Could you check a few things on this model? Use its own coordinates, in mm. Give positions to 0.01 mm unless a question says otherwise; leave off trailing zeros. Write each loop counter-clockwise with the first axis right and the second up, starting at its lowest first coordinate (ties: lowest second). Pieces come first, ordered by that corner, then holes. Notation, with made-up numbers: (-13.5, 8.5) -> (35.5, 8.5) arc R7 ccw to (35.5, 13.5) -> close; hole circle Ø1 at (24.25, -24). An arc over 180 degrees is marked (long way). Write item = value, one per line. Start each with the question number.
```python
from build123d import *

# Parameters (mm, degrees)
SKETCH_1_W      = 26.5
SKETCH_1_H      = 21
SKETCH_1_R      = 0.4
EXTRUDE_1_DEPTH = 1.6
SKETCH_2_W      = 5.5
SKETCH_2_H      = 10
EXTRUDE_2_DEPTH = 1.6


with BuildPart() as part:
    # Эскиз1 → Бобышка-Вытянуть1 (new body)
    with BuildSketch(Plane.XY):
        Rectangle(SKETCH_1_W, SKETCH_1_H)
        with Locations((-11.43, -9)):
            Circle(SKETCH_1_R, mode=Mode.SUBTRACT)
        with Locations((-8.89, -9)):
            Circle(SKETCH_1_R, mode=Mode.SUBTRACT)
        with Locations((-6.35, -9)):
            Circle(SKETCH_1_R, mode=Mode.SUBTRACT)
        with Locations((-3.81, -9)):
            Circle(SKETCH_1_R, mode=Mode.SUBTRACT)
        with Locations((-1.27, -9)):
            Circle(SKETCH_1_R, mode=Mode.SUBTRACT)
        with Locations((1.27, -9)):
            Circle(SKETCH_1_R, mode=Mode.SUBTRACT)
        with Locations((3.81, -9)):
            Circle(SKETCH_1_R, mode=Mode.SUBTRACT)
        with Locations((6.35, -9)):
            Circle(SKETCH_1_R, mode=Mode.SUBTRACT)
        with Locations((8.89, -9)):
            Circle(SKETCH_1_R, mode=Mode.SUBTRACT)
        with Locations((11.43, -9)):
            Circle(SKETCH_1_R, mode=Mode.SUBTRACT)
        with Locations((-11.43, 9)):
            Circle(SKETCH_1_R, mode=Mode.SUBTRACT)
        with Locations((-8.89, 9)):
            Circle(SKETCH_1_R, mode=Mode.SUBTRACT)
        with Locations((-6.35, 9)):
            Circle(SKETCH_1_R, mode=Mode.SUBTRACT)
        with Locations((-3.81, 9)):
            Circle(SKETCH_1_R, mode=Mode.SUBTRACT)
        with Locations((-1.27, 9)):
            Circle(SKETCH_1_R, mode=Mode.SUBTRACT)
        with Locations((1.27, 9)):
            Circle(SKETCH_1_R, mode=Mode.SUBTRACT)
        with Locations((3.81, 9)):
            Circle(SKETCH_1_R, mode=Mode.SUBTRACT)
        with Locations((6.35, 9)):
            Circle(SKETCH_1_R, mode=Mode.SUBTRACT)
        with Locations((8.89, 9)):
            Circle(SKETCH_1_R, mode=Mode.SUBTRACT)
        with Locations((11.43, 9)):
            Circle(SKETCH_1_R, mode=Mode.SUBTRACT)
        with Locations((-8.89, 6.46)):
            Circle(SKETCH_1_R, mode=Mode.SUBTRACT)
        with Locations((-6.35, 6.46)):
            Circle(SKETCH_1_R, mode=Mode.SUBTRACT)
        with Locations((-3.81, 6.46)):
            Circle(SKETCH_1_R, mode=Mode.SUBTRACT)
        with Locations((-1.27, 6.46)):
            Circle(SKETCH_1_R, mode=Mode.SUBTRACT)
        with Locations((1.27, 6.46)):
            Circle(SKETCH_1_R, mode=Mode.SUBTRACT)
        with Locations((3.81, 6.46)):
            Circle(SKETCH_1_R, mode=Mode.SUBTRACT)
        with Locations((6.35, 6.46)):
            Circle(SKETCH_1_R, mode=Mode.SUBTRACT)
        with Locations((8.89, 6.46)):
            Circle(SKETCH_1_R, mode=Mode.SUBTRACT)
        with Locations((11.43, 6.46)):
            Circle(SKETCH_1_R, mode=Mode.SUBTRACT)
        with Locations((-11.43, 6.46)):
            Circle(SKETCH_1_R, mode=Mode.SUBTRACT)
    extrude(amount=EXTRUDE_1_DEPTH)

    # Эскиз2 → Бобышка-Вытянуть2 (add)
    with BuildSketch(Plane.XY.offset(1.6)):
        Rectangle(SKETCH_2_W, SKETCH_2_H)
    extrude(amount=EXTRUDE_2_DEPTH)


solid = part.part
```
(1) We'd pull the mould along Y, two halves only. Please class faces 1 (the flat face through (0, -10.5, 1)), 2 (the flat face through (2.75, 0, 2)), 3 (the cylindrical face through (11.11, -9.24, 0.79)): released by +Y, released by -Y, zero draft, split by the parting line, or undercut.
(2) Imagine slicing it at C-C (y = 6.46). State how many separate pieces and enclosed holes the cut face has, then the cut area to 3 significant figures.
(3) Imagine slicing it at A-A (x = -8.89). Please give me the cut outline in (y, z).
(4) I'm going to push flat-ended pins straight in: pin 1 (0.8 mm diameter, centred on y = 1.5, z = 2.5, fed in from -X); pin 2 (1.3 mm diameter, centred on x = 1, z = 2, fed in from -Y); pin 3 (12 mm diameter, centred on x = 10, y = -4, fed in from +Z); pin 4 (1.5 mm diameter, centred on y = -3.5, z = 2.5, fed in from +X). Where does each tip first touch, or does it pass through?
(5) Imagine slicing it at B-B (x = 2.25). Please give me the cut outline in (y, z).
(6) If I drill on line 1 along Y through (x, z) = (-6.35, 0.55); line 2 along Y through (x, z) = (1, 1.1); line 3 along Z through (x, y) = (-7, -7.5), over which ranges is the centre line in solid material (lowest first)? Write a range as from..to.
(7) Imagine slicing it at D-D (z = 2.55). Please give me the cut outline in (x, y), then the cut area to 3 significant figures.
Answers below:
q1.face_1 = released by -Y
q1.face_2 = zero draft
q1.face_3 = undercut
q2.separate_pieces = 11
q2.enclosed_holes = 0
q2.area = 29.6 mm^2
q3.outline = (-10.5, 0) -> (-9.4, 0) -> (-9.4, 1.6) -> (-10.5, 1.6) -> close; (-8.6, 0) -> (6.06, 0) -> (6.06, 1.6) -> (-8.6, 1.6) -> close; (6.86, 0) -> (8.6, 0) -> (8.6, 1.6) -> (6.86, 1.6) -> close; (9.4, 0) -> (10.5, 0) -> (10.5, 1.6) -> (9.4, 1.6) -> close
q4.pin_1 = -2.75
q4.pin_2 = -10.5
q4.pin_3 = 1.6
q4.pin_4 = 2.75
q5.outline = (-10.5, 0) -> (10.5, 0) -> (10.5, 1.6) -> (5, 1.6) -> (5, 3.2) -> (-5, 3.2) -> (-5, 1.6) -> (-10.5, 1.6) -> close
q6.line_1 = -10.5..-9.4, -8.6..6.06, 6.86..8.6, 9.4..10.5
q6.line_2 = -10.5..-9.3, -8.7..6.16, 6.76..8.7, 9.3..10.5
q6.line_3 = 0..1.6
q7.outline = (-2.75, -5) -> (2.75, -5) -> (2.75, 5) -> (-2.75, 5) -> close
q7.area = 55.0 mm^2
